Work out the finished part from the listing and answer in its coordinate system (mm). A direction names the side the tool comes from. Round coordinates to 2 decimals unless told otherwise and drop trailing zeros. Loops run counter-clockwise (first coordinate to the right, second up) from the corner with the lowest first, then second, coordinate; pieces in that order, holes last.
```python
from build123d import *

# Parameters (mm, degrees)
SKETCH1_R          = 3.96875
EXTRUDE1_DEPTH     = 38.1
CUT_EXTRUDE1_DEPTH = 60.67726868
CUT_EXTRUDE2_START = -38.1
SKETCH3_R          = 6.5405
CUT_EXTRUDE2_DEPTH = 11.43
SKETCH4_W          = 7.9248
SKETCH4_H          = 7.9248
EXTRUDE2_DEPTH     = 2.54


with BuildPart() as part:
    # Sketch1 → Extrude1 (new body)
    with BuildSketch(Plane.XY):
        with BuildLine():
            Line((-12.445441008, 4.399037801), (-12.445441008, -14.650962199))
            Line((-12.445441008, -14.650962199), (25.654558992, -14.650962199))
            Line((25.654558992, -14.650962199), (25.654558992, 4.399037801))
            ThreePointArc((25.654558992, 4.399037801), (6.604558992, 23.449037801), (-12.445441008, 4.399037801))
        make_face()
        with Locations(Location((6.604558992, 4.399037801, 0), (0, 0, 180))):
            Circle(SKETCH1_R, mode=Mode.SUBTRACT)
    extrude(amount=EXTRUDE1_DEPTH)

    # Sketch2 → Cut-Extrude1 (cut, through all)
    with BuildSketch(Plane.XZ.offset(14.650962199)):
        with BuildLine():
            ThreePointArc((10.770158992, 19.05), (9.550083, 21.995524008), (6.604558992, 23.2156))
            Line((6.604558992, 23.2156), (6.604558992, 14.8844))
            ThreePointArc((6.604558992, 14.8844), (9.550083, 16.104475992), (10.770158992, 19.05))
        make_face()
        with BuildLine():
            Line((6.604558992, 14.8844), (6.604558992, 23.2156))
            ThreePointArc((6.604558992, 23.2156), (2.438958992, 19.05), (6.604558992, 14.8844))
        make_face()
    extrude(amount=-CUT_EXTRUDE1_DEPTH, mode=Mode.SUBTRACT)

    # Sketch3 → Cut-Extrude2 (cut)
    with BuildSketch(Plane.XZ.offset(14.650962199).offset(CUT_EXTRUDE2_START)):
        with Locations(Location((6.604558992, 19.05, 0), (0, 0, 90))):
            Circle(SKETCH3_R)
    extrude(amount=CUT_EXTRUDE2_DEPTH, mode=Mode.SUBTRACT)

    # Sketch4 → Extrude2 (add)
    with BuildSketch(Plane.XZ.offset(14.650962199)):
        with Locations((-8.483041008, 19.05)):
            Rectangle(SKETCH4_W, SKETCH4_H)
        with Locations((21.692158992, 19.05)):
            Rectangle(SKETCH4_W, SKETCH4_H)
    extrude(amount=EXTRUDE2_DEPTH)


solid = part.part
```
1. Find section A-A (y = -9.5). Write down the section's boundary in (x, z), then the cut area to 3 significant figures.
Answer key:
outline: (-12.45, 0) - (25.65, 0) - (25.65, 38.1) - (-12.45, 38.1) - close; hole circle Ø8.33 at (6.6, 19.05)
area: 1,400 mm2
2. Given pin 1 (0.8 mm diameter, centred on x = -7, y = -16, fed in from +Z); pin 2 (7 mm diameter, centred on x = 6.6, y = 4.4, fed in from -Z); pin 3 (0.8 mm diameter, centred on x = 20, y = -16, fed in from -Z); pin 4 (4 mm diameter, centred on x = 8, z = 22, fed in from +Y), each flat-ended and moving along its own axis, determine where each tip first touches the part or whether it passes through.
Answer key:
pin 1: stops at z = 23.01
pin 2: passes through
pin 3: stops at z = 15.09
pin 4: stops at y = 12.02
3. Find section C-C (x = 8). Write down the section's boundary in (y, z).
Answer key:
outline: (-14.65, 0) - (0.68, 0) - (0.68, 15.13) - (-14.65, 15.13) - close; (-14.65, 22.97) - (0.68, 22.97) - (0.68, 38.1) - (-14.65, 38.1) - close; (8.11, 0) - (23.4, 0) - (23.4, 12.66) - (12.02, 12.66) - (12.02, 15.13) - (8.11, 15.13) - close; (8.11, 22.97) - (12.02, 22.97) - (12.02, 25.44) - (23.4, 25.44) - (23.4, 38.1) - (8.11, 38.1) - close
4. Consider probe 1 along X at (y, z) = (14.75, 19.05); probe 2 along X at (y, z) = (5.5, 5); probe 3 along Y at (x, z) = (10, 22). Determine where each line is inside the solid, lowest interval first.
Answer key:
probe 1: x = -9.39 to 0.06, 13.15 to 22.6
probe 2: x = -12.41 to 2.79, 10.42 to 25.62
probe 3: y = -14.65 to 2.34, 6.45 to 12.02
5. Find section B-B (z = 35). Write down the section's boundary in (x, y).
Answer key:
outline: (-12.45, -14.65) - (25.65, -14.65) - (25.65, 4.4) arc R19.05 ccw to (-12.45, 4.4) - close; hole circle Ø7.94 at (6.6, 4.4)
6. Find section D-D (x = 23.5). Write down the section's boundary in (y, z).
Answer key:
outline: (-17.19, 15.09) - (-14.65, 15.09) - (-14.65, 0) - (13.2, 0) - (13.2, 38.1) - (-14.65, 38.1) - (-14.65, 23.01) - (-17.19, 23.01) - close
7. Determine the mould class of faces 4 (the face through (-9, -17.191, 19)), 5 (the face through (6, 0, 38.1)), 6 (the face through (4.77, 7.92, 29.08)) for opening direction Y: +Y half, -Y half, draft (parallel to the pull), parting line (faces both ways), or undercut.
Answer key:
face 4: -Y half
face 5: draft
face 6: undercut
8. Which of the six approach directions +Z, -Z, +X, -X, +Y, -Y give full straight-line access (tool end or side, diameter ignored) to faces 1 (the face through (6.317, 17.814, 12.516)), 2 (the face through (22, -16, 15.088)), 3 (the face through (-4.521, -16, 19))?
Answer key:
face 1: +Y
face 2: -Z, +X, -X, -Y
face 3: +Z, -Z, -Y
